Model file for the job. Use its own axes, mm. A direction names the side the tool comes from. Round coordinates to 2 decimals unless told otherwise and drop trailing zeros. Order: outer loops, then holes, each group sorted by start corner. A loop starts at its lowest first (then second) coordinate and runs counter-clockwise, first axis right, second up. Notation, with made-up numbers: (27, 37) -> (44, 37) arc R13 ccw to (44, 62) -> close; hole circle Ø4 at (5.25, -11). An arc over 180 degrees is marked (long way). Put each result on its own line as item: value. Start each with the question number.
Q1. 3-axis set-ups, long thin cutter, end or side, ignore diameter. For faces 1 (the face through (-2.09, -46.64, -1.61)), 2 (the face through (-4.51, -43.36, 38.39)), 3 (the face through (-4.96, -50.92, 41.61)), 4 (the face through (-4.51, -43.36, -1.61)), 5 (the face through (-4.96, -5.92, 41.61)): which of +Z, -Z, +X, -X, +Y, -Y reach the whole face in a straight line?
Q2. Cut at D-D, the plane x = 1.5. List the corners of the cut face in (y, z), and give its area (3 significant figures).
Q3. Probe L1, parallel to X at y = -3, z = 36.5; L2, parallel to Y at x = 0.5, z = 39; L3, parallel to Z at x = 6.25, y = -14.5. List the from-to ranges inside material, lowest first.
Q4. Cut at A-A, the plane y = -3. State how many separate pieces and enclosed holes the cut face has, and give its area (3 significant figures).
Q5. Cut at B-B, the plane z = 12.75. List the corners of the cut face in (x, y), and give its area (3 significant figures).
Q6. Pull direction Y, two halves, no side cores. Call faces 6 (the face through (-1.64, -22.81, -1.61)), 7 (the face through (-8.24, -4.95, -1.61)), 8 (the face through (1, -47.3, 20)): released by +Y, released by -Y, zero draft, split by the parting line, or undercut.
Q7. Flat gauge pins, fed straight in: P1, Ø20, axis at y = -27, z = 15.5, coming from the +X side; P2, Ø1, axis at y = -6, z = 2.5, coming from the -X side; P3, Ø2, axis at x = 4.5, z = 15, coming from the -Y side. Where does each tip first touch, or does it go through?
from build123d import *

# Parameters (mm, degrees)
EXTRU_MINCE1_DEPTH         = 2.3
CONG_1_R                   = 2.3
ESQUISSE2_W                = 40
ESQUISSE2_H                = 49.6
BOSS_EXTRU_1_DEPTH         = 2.3
R_P_TITION_LIN_AIRE1_COUNT = 2
R_P_TITION_LIN_AIRE1_PITCH = 40
CONG_2_R                   = 2.3
ESQUISSE3_R                = 3.25
BOSS_EXTRU_2_DEPTH         = 12
CONG_3_R                   = 3.25


with BuildPart() as part:
    # Esquisse1 → Extru.-Mince1 (new, symmetric)
    with BuildSketch(Plane.XY):
        Polygon((-4.3, -57), (-4.3, -47.3), (2.3, -47.3), (2.3, 2.3), (-8.9, 2.3), (-8.9, -12), (-4.3, -12), (-4.3, -2.3), (-2.3, -2.3), (-2.3, -42.7), (-8.9, -42.7), (-8.9, -57), align=None)
    extru_mince1 = extrude(amount=EXTRU_MINCE1_DEPTH, both=True)

    # Congé1
    cong_1_edges = [part.edges().sort_by_distance(p)[0] for p in [
        (-6.6, -57, -2.3),
        (-4.3, -52.15, -2.3),
        (-1, -47.3, -2.3),
        (2.3, -22.5, -2.3),
        (-3.3, 2.3, -2.3),
        (-8.9, -4.85, -2.3),
        (-6.6, -12, -2.3),
        (-4.3, -7.15, -2.3),
        (-3.3, -2.3, -2.3),
        (-2.3, -22.5, -2.3),
        (-5.6, -42.7, -2.3),
        (-8.9, -49.85, -2.3),
        (-5.6, -42.7, 2.3),
        (-2.3, -22.5, 2.3),
        (-3.3, -2.3, 2.3),
        (-4.3, -7.15, 2.3),
        (-6.6, -12, 2.3),
        (-8.9, -4.85, 2.3),
        (-3.3, 2.3, 2.3),
        (2.3, -22.5, 2.3),
        (-1, -47.3, 2.3),
        (-4.3, -52.15, 2.3),
        (-6.6, -57, 2.3),
        (-8.9, -49.85, 2.3),
    ]]
    fillet(cong_1_edges, radius=CONG_1_R - 0.0001)  # a hair under: the kernel refuses the full size

    # Esquisse2 → Boss.-Extru.1 (add)
    with BuildSketch(Plane(origin=(0, 0, 0), x_dir=(0, 0, -1), z_dir=(1, 0, 0))):
        with Locations((-20, -22.5)):
            Rectangle(ESQUISSE2_W, ESQUISSE2_H)
    extrude(amount=BOSS_EXTRU_1_DEPTH)

    # Répétition linéaire1: Extru.-Mince1 ×2
    with Locations(*[(0, 0, i * R_P_TITION_LIN_AIRE1_PITCH) for i in range(1, R_P_TITION_LIN_AIRE1_COUNT)]):
        add(extru_mince1)

    # Congé2
    cong_2_edges = [part.edges().sort_by_distance(p)[0] for p in [
        (-5.6, -42.7, 42.3),
        (-2.3, -22.5, 42.3),
        (-3.3, -2.3, 42.3),
        (-4.3, -7.15, 42.3),
        (-6.6, -12, 42.3),
        (-8.9, -4.85, 42.3),
        (-3.3, 2.3, 42.3),
        (2.3, -22.5, 42.3),
        (-1, -47.3, 42.3),
        (-4.3, -52.15, 42.3),
        (-6.6, -57, 42.3),
        (-8.9, -49.85, 42.3),
        (-2.15, -47.3, 37.7),
        (-4.3, -52.15, 37.7),
        (-6.6, -57, 37.7),
        (-8.9, -49.85, 37.7),
        (-5.6, -42.7, 37.7),
        (-2.3, -22.5, 37.7),
        (-3.3, -2.3, 37.7),
        (-4.3, -7.15, 37.7),
        (-6.6, -12, 37.7),
        (-8.9, -4.85, 37.7),
        (-4.45, 2.3, 37.7),
    ]]
    fillet(cong_2_edges, radius=CONG_2_R - 0.0001)  # a hair under: the kernel refuses the full size

    # Esquisse3 → Boss.-Extru.2 (add)
    with BuildSketch(Plane(origin=(2.3, 0, 0), x_dir=(0, 0, -1), z_dir=(1, 0, 0))):
        with Locations((-27.25, -17.3)):
            Circle(ESQUISSE3_R)
        with Locations((-12.75, -17.3)):
            Circle(ESQUISSE3_R)
    extrude(amount=BOSS_EXTRU_2_DEPTH)

    # Congé3
    cong_3_edges = [part.edges().sort_by_distance(p)[0] for p in [
        (14.3, -17.3, 30.5),
        (14.3, -17.3, 16),
    ]]
    fillet(cong_3_edges, radius=CONG_3_R)


solid = part.part
Ans:
1. face 1: -Z, +X, -Y
1. face 2: -X
1. face 3: +Z, +X, -Y
1. face 4: -Z, -X
1. face 5: +Z
2. outline: (-47.3, 0) arc R2.3 ccw to (-46.5, -1.74) -> (1.5, -1.74) arc R2.3 ccw to (2.3, 0) -> (2.3, 40) arc R2.3 ccw to (1.5, 41.74) -> (-46.5, 41.74) arc R2.3 ccw to (-47.3, 40) -> close
2. area: 2,160 mm^2
3. L1: x = 0 to 2.3
3. L2: y = -47.3 to 2.3
3. L3: z = 11.1 to 14.4, 25.6 to 28.9
4. separate pieces: 3
4. enclosed holes: 0
4. area: 150 mm^2
5. outline: (0, -47.3) -> (2.3, -47.3) -> (2.3, -20.55) -> (11.05, -20.55) arc R3.25 ccw to (11.05, -14.05) -> (2.3, -14.05) -> (2.3, 2.3) -> (0, 2.3) -> close
5. area: 188 mm^2
6. face 6: undercut
6. face 7: zero draft
6. face 8: released by -Y
7. P1: stops at x = 14.3
7. P2: stops at x = -7.74
7. P3: stops at y = -20.3
